The listing builds one solid part. Answer for the finished solid, in the listing's coordinates (mm). A direction names the side the tool comes from. Give positions to 0.01 mm unless a question says otherwise; leave off trailing zeros. Order: outer loops, then holes, each group sorted by start corner. A loop starts at its lowest first (then second) coordinate and runs counter-clockwise, first axis right, second up. Notation, with made-up numbers: (46, 30.5) - (96, 30.5) arc R16 ccw to (96, 58.5) - close; hole circle Ø8 at (44.25, 49.5). An arc over 180 degrees is marked (long way). Use a Markdown table: item, result. Add a question column.
1) The mould has two halves that part along Z. Classify faces 1 (the face through (25.4, -6, -280)), 2 (the face through (0, -6, -285.986)), 3 (the face through (-215.9, -6, -45)): released by +Z, released by -Z, zero draft, split by the parting line, or undercut.
2) Straight lines are drawn through the part: line 1 (Z direction, x = -149.5, y = -10.25); line 2 (X direction, y = -4, z = -57.5). For each, find the intervals that lie inside material, in ascending order.
3) Find section A-A, the plane y = -9.5. Determine the outline of the cut face in (x, z).
4) Find section C-C, the plane z = -54.5. Determine the outline of the cut face in (x, y).
5) For faces 4 (the face through (-222, -6, -19.286)), 5 (the face through (177.8, -6, -280)), 6 (the face through (222, -6, -19.286)), 7 (the face through (-3, 0, 4)), determine the directions among +Z, -Z, +X, -X, +Y, -Y from which every point of the face is accessible in a straight line to the end or side of a thin tool.
6) Find section B-B, the plane x = -40. Determine the outline of the cut face in (y, z), plus the area to 3 significant figures.
7) Flat-ended cylindrical pins translate along their axes: pin 1 (4 mm diameter, centred on y = -6, z = -42.5, fed in from +X); pin 2 (6.5 mm diameter, centred on x = 107, y = -5.5, fed in from -Z). Find the tip coordinate at first contact, or state that the pin passes through.
from build123d import *

# Parameters (mm, degrees)
F1_DEPTH = 12.7
F2_W     = 12.7
F2_H     = 50.8
F3_DEPTH = 25.4


with BuildPart() as f1:
    # F0 (on Front) → F1 (new body)
    with BuildSketch(Plane.XZ):
        Polygon((25.4, -273.285884), (177.8, -273.285884), (177.8, -285.985884), (228.6, -285.985884), (228.6, -273.285884), (228.6, 285.514116), (-228.6, 285.514116), (-228.6, -273.285884), (-228.6, -285.985884), (-177.8, -285.985884), (-177.8, -273.285884), (-25.4, -273.285884), (-25.4, -285.985884), (25.4, -285.985884), align=None)
    extrude(amount=F1_DEPTH)

    # F2 (on face) → F3 (cut)
    with BuildSketch(Plane.XZ.offset(12.7)):
        with Locations((-222.25, -44.685884)):
            Rectangle(F2_W, F2_H)
        with Locations((222.25, -44.685884)):
            Rectangle(F2_W, F2_H)
    extrude(amount=-F3_DEPTH, mode=Mode.SUBTRACT)


solid = f1.part
The answers:
| question | item | result |
|---|---|---|
| 1 | face 1 | zero draft |
| 1 | face 2 | released by -Z |
| 1 | face 3 | undercut |
| 2 | line 1 | -273.29 to 285.51 |
| 2 | line 2 | -215.9 to 215.9 |
| 3 | outline | (-228.6, -285.99) - (-177.8, -285.99) - (-177.8, -273.29) - (-25.4, -273.29) - (-25.4, -285.99) - (25.4, -285.99) - (25.4, -273.29) - (177.8, -273.29) - (177.8, -285.99) - (228.6, -285.99) - (228.6, -70.09) - (215.9, -70.09) - (215.9, -19.29) - (228.6, -19.29) - (228.6, 285.51) - (-228.6, 285.51) - (-228.6, -19.29) - (-215.9, -19.29) - (-215.9, -70.09) - (-228.6, -70.09) - close |
| 4 | outline | (-215.9, -12.7) - (215.9, -12.7) - (215.9, 0) - (-215.9, 0) - close |
| 5 | face 4 | -X, +Y, -Y |
| 5 | face 5 | -Z, +Y, -Y |
| 5 | face 6 | +X, +Y, -Y |
| 5 | face 7 | +Z, -Z, +X, -X, +Y |
| 6 | outline | (-12.7, -273.29) - (0, -273.29) - (0, 285.51) - (-12.7, 285.51) - close |
| 6 | area | 7,100 mm2 |
| 7 | pin 1 | x = 215.9 |
| 7 | pin 2 | z = -273.29 |
